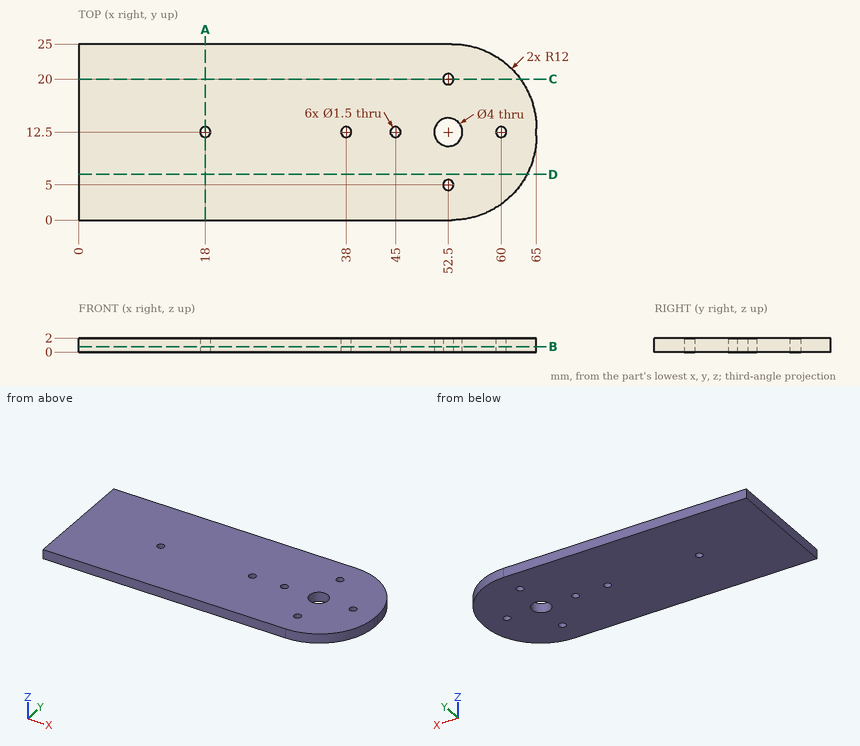
For this review, use the dimensioned drawing (mm, ordinates from the lowest corner) and the shaded views. Round coordinates to 2 decimals unless told otherwise and drop trailing zeros. Write each loop counter-clockwise with the first axis right and the second up, starting at its lowest first coordinate (ties: lowest second). Pieces come first, ordered by that corner, then holes. Notation, with made-up numbers: (60.25, 36.5) - (85.25, 36.5) arc R21 cw to (85.25, 59.5) - close; hole circle Ø8 at (68.5, 84). An arc over 180 degrees is marked (long way). Answer as CSV lines item,"result". Start each with the question number.
(1) We need section A-A on x = 18. State the section outline as (y, z) points.
(2) To check wall thickness, follow line 1 (Y direction, x = 52, z = 1.8); line 2 (Y direction, x = 52.5, z = 0.6); line 3 (X direction, y = 12.75, z = 0.35). State the ranges of each line that lie inside material, in increasing order.
(3) We need section D-D on y = 6.5. State the section outline as (x, z) points.
(4) For pin 1 Ø1.2 at (x, y) = (52.5, 5) entering from -Z, flat-tipped, find the tip position at first contact; note if it passes through.
(5) We need section B-B on z = 0.8. State the section outline as (x, y) points.
(6) We need section C-C on y = 20. State the section outline as (x, z) points.
Worked answers:
1,outline,"(0, 0) - (11.75, 0) - (11.75, 2) - (0, 2) - close; (13.25, 0) - (25, 0) - (25, 2) - (13.25, 2) - close"
2,line 1,"0 to 4.44, 5.56 to 10.56, 14.44 to 19.44, 20.56 to 25"
2,line 2,"0 to 4.25, 5.75 to 10.5, 14.5 to 19.25, 20.75 to 25"
2,line 3,"0 to 17.29, 18.71 to 37.29, 38.71 to 44.29, 45.71 to 50.52, 54.48 to 59.29, 60.71 to 65"
3,outline,"(0, 0) - (63.67, 0) - (63.67, 2) - (0, 2) - close"
4,pin 1,"through"
5,outline,"(0, 0) - (53, 0) arc R12 ccw to (65, 12) - (65, 13) arc R12 ccw to (53, 25) - (0, 25) - close; hole circle Ø1.5 at (18, 12.5); hole circle Ø1.5 at (38, 12.5); hole circle Ø1.5 at (45, 12.5); hole circle Ø4 at (52.5, 12.5); hole circle Ø1.5 at (52.5, 5); hole circle Ø1.5 at (52.5, 20); hole circle Ø1.5 at (60, 12.5)"
6,outline,"(0, 0) - (51.75, 0) - (51.75, 2) - (0, 2) - close; (53.25, 0) - (62.75, 0) - (62.75, 2) - (53.25, 2) - close"
